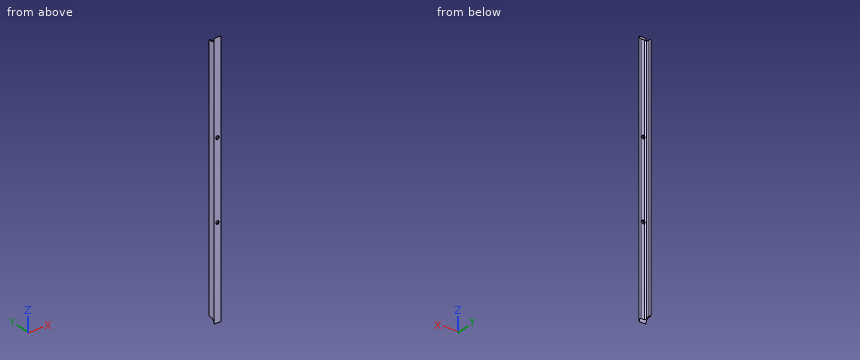
from build123d import *

# Parameters (mm, degrees)
MIEMBRO_ESTRUCTURAL1_DEPTH    = 780.7
CORTAR_EXTRUIR2_DEPTH         = 600.996074077
TALADRO_DE_MARGEN_PARA_3_81_D = 10.0838


with BuildPart() as part:
    # Sketch1 → Miembro estructural1 (new body)
    with BuildSketch(Plane.XY.offset(-599.329032258)):
        with BuildLine():
            Line((0, 0), (0, 20))
            ThreePointArc((0, 20), (2.121320344, 19.121320344), (3, 17))
            Line((3, 17), (3, 6.5))
            ThreePointArc((3, 6.5), (4.025126266, 4.025126266), (6.5, 3))
            Line((6.5, 3), (17, 3))
            ThreePointArc((17, 3), (19.121320344, 2.121320344), (20, 0))
            Line((20, 0), (0, 0))
        make_face()
    extrude(amount=MIEMBRO_ESTRUCTURAL1_DEPTH)

    # Croquis2 → Cortar-Extruir2 (cut, through all)
    with BuildSketch(Plane.YZ):
        with BuildLine():
            Line((20, 181.370967742), (0, 181.370967742))
            ThreePointArc((0, 181.370967742), (3.743979256, 172.325057712), (12.785701293, 168.570975728))
            Line((12.785701293, 168.570975728), (20, 168.570975728))
            Line((20, 168.570975728), (20, 181.370967742))
        make_face()
        with BuildLine():
            ThreePointArc((12.785701293, -586.529040245), (3.743979256, -590.283122228), (0, -599.329032258))
            Line((0, -599.329032258), (20, -599.329032258))
            Line((20, -599.329032258), (20, -586.529040245))
            Line((20, -586.529040245), (12.785701293, -586.529040245))
        make_face()
    extrude(amount=CORTAR_EXTRUIR2_DEPTH, mode=Mode.SUBTRACT)

    # Taladro de margen para 3/81 (through all)
    with Locations(Plane(origin=(0, 0, 0), x_dir=(-1, 0, 0), z_dir=(0, -1, 0))):
        with Locations((-10, 92.979032258), (-10, 324.979032258)):
            Hole(TALADRO_DE_MARGEN_PARA_3_81_D / 2)


solid = part.part
Can you work these out from the model? Positions are in its coordinate system, mm. Coordinates: 2 decimals unless noted, no trailing zeros. Write each loop counter-clockwise with the first axis right and the second up, starting at its lowest first coordinate (ties: lowest second). Pieces come first, ordered by that corner, then holes.
Q1. Imagine slicing it at B-B, the plane z = -171. List the corners of the cut face in (x, y) for me.
Results found:
outline: (0, 0) - (20, 0) arc R3 ccw to (17, 3) - (6.5, 3) arc R3.5 cw to (3, 6.5) - (3, 17) arc R3 ccw to (0, 20) - close
Q2. For P1, Ø3, axis at y = 18, z = 24, coming from the +X side; P2, Ø0.9, axis at x = 1.5, y = 15, coming from the +Z side; P3, Ø10, axis at x = 13.5, y = 6, coming from the +Z side, each with a flat end and sliding along its axis, tell me the tip position at first contact or that it passes through.
Results found:
P1: stops at x = 3
P2: stops at z = 168.57
P3: stops at z = 176.41
Q3. Imagine slicing it at A-A, the plane x = 10. List the corners of the cut face in (y, z) for me.
Results found:
outline: (0, -599.33) arc R12.8 cw to (3, -591.09) - (3, -330.02) - (0, -330.02) - close; (0, -319.94) - (3, -319.94) - (3, -98.02) - (0, -98.02) - close; (0, -87.94) - (3, -87.94) - (3, 173.14) arc R12.8 cw to (0, 181.37) - close
Q4. Please list where these lines run through material, in increasing order: L1, parallel to Z at x = 10, y = 2.1; L2, parallel to X at y = 16.25, z = -270.5; L3, parallel to Z at x = 10, y = 2.
Results found:
L1: z = -592.3 to -330.02, -319.94 to -98.02, -87.94 to 174.35
L2: x = 0 to 3
L3: z = -592.46 to -330.02, -319.94 to -98.02, -87.94 to 174.5
